Read the model definition and answer for the solid it produces. Units are mm, in the model's axes. Give positions to 0.01 mm unless a question says otherwise; leave off trailing zeros. Order: outer loops, then holes, each group sorted by start corner. A loop starts at its lowest first (then second) coordinate and runs counter-clockwise, first axis right, second up. Notation, with made-up numbers: (-21.75, 29.25) -> (35.25, 29.25) arc R28 ccw to (35.25, 49.25) -> close; hole circle Ø1 at (48.25, -32.75). An arc over 180 degrees is marked (long way). Use one line per item in the form item = value.
```python
from build123d import *

# Parameters (mm, degrees)
F1_DEPTH = 6.35
F2_R     = 1.5875
F3_DEPTH = 6.35


with BuildPart() as f1:
    # F0 (on Top) → F1 (new body)
    with BuildSketch(Plane.XY):
        with BuildLine():
            ThreePointArc((-1.8402014017, 18.9609113389), (-22.248244758, 22.6512274543), (-18.9248270392, 2.1802342852))
            ThreePointArc((-18.9248270392, 2.1802342852), (-13.3489468548, 13.5907364726), (-1.8402014017, 18.9609113389))
        make_face()
        with BuildLine():
            ThreePointArc((-1.8402014017, 18.9609113389), (-13.3489468548, 13.5907364726), (-18.9248270392, 2.1802342852))
            ThreePointArc((-18.9248270392, 2.1802342852), (-6.6230148875, 2.8180005541), (-0.6489468548, 13.5907364726))
            ThreePointArc((-0.6489468548, 13.5907364726), (-0.9503367058, 16.3410939716), (-1.8402014017, 18.9609113389))
        make_face()
        with BuildLine():
            ThreePointArc((2.1802342852, 18.9248270392), (4.5302454909, 4.4496489516), (18.9609113389, 1.8402014017))
            ThreePointArc((18.9609113389, 1.8402014017), (13.5907364726, 13.3489468548), (2.1802342852, 18.9248270392))
        make_face()
        with BuildLine():
            ThreePointArc((2.1802342852, 18.9248270392), (13.5907364726, 13.3489468548), (18.9609113389, 1.8402014017))
            ThreePointArc((18.9609113389, 1.8402014017), (24.3026742245, 6.5266019794), (26.2907364726, 13.3489468548))
            ThreePointArc((26.2907364726, 13.3489468548), (16.4522589886, 25.7223735786), (2.1802342852, 18.9248270392))
        make_face()
        with BuildLine():
            ThreePointArc((-18.9248270392, 2.1802342852), (-1.0919122914, -19.0186810149), (19.05, 0))
            ThreePointArc((19.05, 0), (19.0277147998, 0.9211783199), (18.9609113389, 1.8402014017))
            ThreePointArc((18.9609113389, 1.8402014017), (4.5302454909, 4.4496489516), (2.1802342852, 18.9248270392))
            ThreePointArc((2.1802342852, 18.9248270392), (0.1709710784, 19.0492327638), (-1.8402014017, 18.9609113389))
            ThreePointArc((-1.8402014017, 18.9609113389), (-0.9503367058, 16.3410939716), (-0.6489468548, 13.5907364726))
            ThreePointArc((-0.6489468548, 13.5907364726), (-6.6230148875, 2.8180005541), (-18.9248270392, 2.1802342852))
        make_face()
    extrude(amount=F1_DEPTH)

    # F2 (on face) → F3 (cut, through all)
    with BuildSketch(Plane(origin=(0, 0, 0), x_dir=(1, 0, 0), z_dir=(0, 0, -1))):
        with Locations((0, 10.0062619895)):
            Circle(F2_R)
    extrude(amount=-F3_DEPTH, mode=Mode.SUBTRACT)


solid = f1.part
```
Item 1: The part is cut by section D-D on x = -14.5. Give the vertices of the cut face in (y, z), and give its area (3 significant figures).
Checks:
outline = (-12.36, 0) -> (26.24, 0) -> (26.24, 6.35) -> (-12.36, 6.35) -> close
area = 245 mm²
Item 2: Straight lines are drawn through the part: L1, parallel to Y at x = 0, z = 2.25; L2, parallel to X at y = 20, z = 5.25; L3, parallel to X at y = -11, z = 2. For each, find the intervals that lie inside material, in ascending order. Write a range as from..to.
Checks:
L1 = -19.05..-11.59, -8.42..19.05
L2 = -24.31..-2.38, 2.77..24.41
L3 = -15.55..-1.24, 1.24..15.55
Item 3: Determine the mould class of faces 1 (the flat face through (0, 4, 6.35)), 2 (the cylindrical face through (0.2, 19.05, 3.13)) for opening direction X: +X half, -X half, draft (parallel to the pull), parting line (faces both ways), or undercut.
Checks:
face_1 = draft
face_2 = undercut
Item 4: The part is cut by section A-A on x = 0. Give the vertices of the cut face in (y, z), and give its area (3 significant figures).
Checks:
outline = (-19.05, 0) -> (-11.59, 0) -> (-11.59, 6.35) -> (-19.05, 6.35) -> close; (-8.42, 0) -> (19.05, 0) -> (19.05, 6.35) -> (-8.42, 6.35) -> close
area = 222 mm²
Item 5: Given pin 1 Ø1.5 at (y, z) = (21.5, 3) entering from -X; pin 2 Ø3 at (y, z) = (18, 5) entering from +X; pin 3 Ø1.5 at (x, z) = (3.5, 1.5) entering from -Y, each flat-ended and moving along its own axis, determine where each tip first touches the part or whether it passes through.
Checks:
pin_1 = -23.84
pin_2 = 25.89
pin_3 = -18.85
Item 6: The part is cut by section C-C on y = 18. Give the vertices of the cut face in (x, z), and give its area (3 significant figures).
Checks:
outline = (-25.26, 0) -> (25.41, 0) -> (25.41, 6.35) -> (-25.26, 6.35) -> close
area = 322 mm²
